Design review of the part built by this model. Coordinates are the model's own, in mm. Face numbers are marked on the shaded views. A direction names the side the tool comes from. Coordinates: 2 decimals unless noted, no trailing zeros. Loops run counter-clockwise (first coordinate to the right, second up) from the corner with the lowest first, then second, coordinate; pieces in that order, holes last. Notation, with made-up numbers: M 87.5,7 L 139.5,7 A32 cw 139.5,40 Z; hole C -37,-31.5 d1. An arc over 180 degrees is marked long. Put each result on its own line as item: value. Start each with the question number.
(1) Clearance check with flat-ended pins moving along their axes: pin 1 (6 mm diameter, centred on x = -30, y = 3, fed in from +Z); pin 2 (3.5 mm diameter, centred on x = -2, y = 1, fed in from +Z); pin 3 (2.5 mm diameter, centred on x = -20.5, z = 3.5, fed in from +Y); pin 4 (1.6 mm diameter, centred on x = 28.975, y = 11.475, fed in from +Z). State where each tip first meets the part, or that it passes through.
(2) Take a section at A-A, the plane z = 2.1. Give the boundary of the cut face in (x, y).
(3) Take a section at C-C, the plane y = 0.5. Give the boundary of the cut face in (x, z), then the cut area to 3 significant figures.
(4) For probe 1 along X at (y, z) = (0.5, 1.85); probe 2 along X at (y, z) = (-12.5, 4.1); probe 3 along Y at (x, z) = (-24.5, 2.3), list the stretches that pass through material, from the lowest coordinate up. Write a range as [from, to].
(5) For the marked faces 1, 2, 3 and 4, list the 3-axis set-ups (+Z, -Z, +X, -X, +Y, -Y) from which the entire face can be reached by the end or side of a thin tool; tool diameter is ignored.
(6) Take a section at D-D, the plane x = -22. Give the boundary of the cut face in (y, z), then the cut area to 3 significant figures.
(7) Take a section at B-B, the plane x = -1. Give the boundary of the cut face in (y, z), then the cut area to 3 significant figures.
(8) The part is to be moulded in two halves that separate along X. For the marked faces 5 and 6, say which applies: +X half, -X half, draft (parallel to the pull), parting line (faces both ways), or undercut.
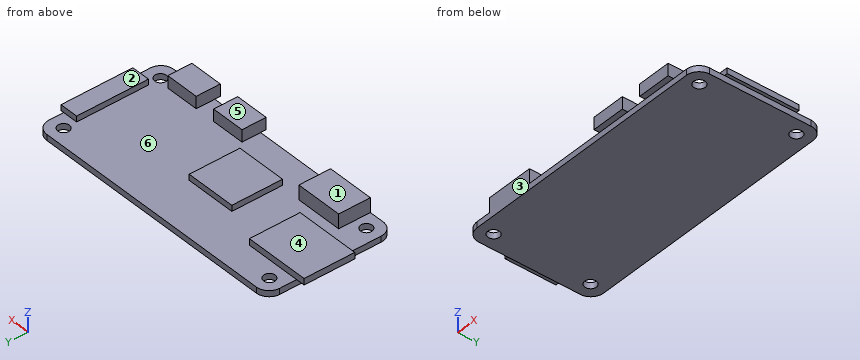
```python
from build123d import *

# Parameters (mm, degrees)
F0_R     = 1.375
F1_DEPTH = 1.4
F2_W     = 12
F2_H     = 12
F3_DEPTH = 1.4
F2_W_2   = 11.2
F2_H_2   = 7.5
F4_DEPTH = 3.4
F2_W_3   = 8
F2_H_3   = 4.4
F2_H_4   = 1.3
F5_DEPTH = 2.85
F2_W_4   = 3.65
F2_H_5   = 17
F2_W_5   = 0.75
F6_DEPTH = 1.35
F2_W_6   = 2.1
F2_W_7   = 13.3
F7_DEPTH = 1.5


with BuildPart() as f1:
    # F0 (on Top) → F1 (new body)
    with BuildSketch(Plane.XY):
        with BuildLine():
            Line((-29.5, -15), (29.5, -15))
            ThreePointArc((29.5, -15), (31.62132, -14.12132), (32.5, -12))
            Line((32.5, -12), (32.5, 12))
            ThreePointArc((32.5, 12), (31.62132, 14.12132), (29.5, 15))
            Line((29.5, 15), (-29.5, 15))
            ThreePointArc((-29.5, 15), (-31.62132, 14.12132), (-32.5, 12))
            Line((-32.5, 12), (-32.5, -12))
            ThreePointArc((-32.5, -12), (-31.62132, -14.12132), (-29.5, -15))
        make_face()
        with Locations((-28.975, -11.475)):
            Circle(F0_R, mode=Mode.SUBTRACT)
        with Locations((28.975, -11.475)):
            Circle(F0_R, mode=Mode.SUBTRACT)
        with Locations((-28.975, 11.475)):
            Circle(F0_R, mode=Mode.SUBTRACT)
        with Locations((28.975, 11.475)):
            Circle(F0_R, mode=Mode.SUBTRACT)
    extrude(amount=F1_DEPTH)

    # F2 (on face) → F3 (join)
    with BuildSketch(Plane.XY.offset(1.4)):
        with Locations((-3.5, -2)):
            Rectangle(F2_W, F2_H)
    extrude(amount=F3_DEPTH)

    # F2 (on face) → F4 (join)
    with BuildSketch(Plane.XY.offset(1.4)):
        with Locations((-20.3, -11.25)):
            Rectangle(F2_W_2, F2_H_2)
    extrude(amount=F4_DEPTH)

    # F2 (on face) → F5 (join)
    with BuildSketch(Plane.XY.offset(1.4)):
        with Locations((9, -12.8)):
            Rectangle(F2_W_3, F2_H_3)
        with Locations((21.9, -12.8)):
            Rectangle(F2_W_3, F2_H_3)
        with Locations((21.9, -15.65)):
            Rectangle(F2_W_3, F2_H_4)
        with Locations((9, -15.65)):
            Rectangle(F2_W_3, F2_H_4)
    extrude(amount=F5_DEPTH)

    # F2 (on face) → F6 (join)
    with BuildSketch(Plane.XY.offset(1.4)):
        with Locations((30.675, 0)):
            Rectangle(F2_W_4, F2_H_5)
        with Locations((32.875, 0)):
            Rectangle(F2_W_5, F2_H_5)
    extrude(amount=F6_DEPTH)

    # F2 (on face) → F7 (join)
    with BuildSketch(Plane.XY.offset(1.4)):
        with Locations((-33.55, 2)):
            Rectangle(F2_W_6, F2_H)
        with Locations((-25.85, 2)):
            Rectangle(F2_W_7, F2_H)
    extrude(amount=F7_DEPTH)


solid = f1.part
```
Computed values:
1. pin 1: stops at z = 2.9
1. pin 2: stops at z = 2.8
1. pin 3: stops at y = 8
1. pin 4: passes through
2. outline: M -34.6,-4 L -19.2,-4 L -19.2,8 L -34.6,8 Z; M -25.9,-15 L -14.7,-15 L -14.7,-7.5 L -25.9,-7.5 Z; M -9.5,-8 L 2.5,-8 L 2.5,4 L -9.5,4 Z; M 5,-16.3 L 13,-16.3 L 13,-10.6 L 5,-10.6 Z; M 17.9,-16.3 L 25.9,-16.3 L 25.9,-10.6 L 17.9,-10.6 Z; M 28.85,-8.5 L 33.25,-8.5 L 33.25,8.5 L 28.85,8.5 Z
3. outline: M -34.6,1.4 L -32.5,1.4 L -32.5,0 L 32.5,0 L 32.5,1.4 L 33.25,1.4 L 33.25,2.75 L 28.85,2.75 L 28.85,1.4 L 2.5,1.4 L 2.5,2.8 L -9.5,2.8 L -9.5,1.4 L -19.2,1.4 L -19.2,2.9 L -34.6,2.9 Z
3. area: 137 mm^2
4. probe 1: x = [-34.6, -19.2], [-9.5, 2.5], [28.85, 33.25]
4. probe 2: x = [-25.9, -14.7], [5, 13], [17.9, 25.9]
4. probe 3: y = [-15, -7.5], [-4, 8]
5. face 1: +Z, +X, -X, +Y, -Y
5. face 2: +Z, +X, +Y, -Y
5. face 3: -Z, -X, -Y
5. face 4: +Z, +X, -X, +Y
6. outline: M -15,0 L 15,0 L 15,1.4 L 8,1.4 L 8,2.9 L -4,2.9 L -4,1.4 L -7.5,1.4 L -7.5,4.8 L -15,4.8 Z
6. area: 85.5 mm^2
7. outline: M -15,0 L 15,0 L 15,1.4 L 4,1.4 L 4,2.8 L -8,2.8 L -8,1.4 L -15,1.4 Z
7. area: 58.8 mm^2
8. face 5: draft
8. face 6: undercut
